Model file for the job. Use its own axes, mm. A direction names the side the tool comes from. Coordinates: 2 decimals unless noted, no trailing zeros. Loops run counter-clockwise (first coordinate to the right, second up) from the corner with the lowest first, then second, coordinate; pieces in that order, holes last.
from build123d import *

# Parameters (mm, degrees)
EXTRUDE_1_DEPTH = 15
FILLET_1_R      = 2
FILLET_2_R      = 2.5


# Read off the part's stored shape, not the designer's step: Отверстие с зазором M41
with BuildPart() as part:
    # Эскиз1 → Бобышка-Вытянуть1 (new body)
    with BuildSketch(Plane(origin=(0, 0, 0), x_dir=(1, 0, 0), z_dir=(0, 1, 0))):
        with BuildLine():
            Line((-22.5, -46.880166382), (-22.5, -45.768438907))
            ThreePointArc((-22.5, -45.768438907), (-17.354305588, -47.956522784), (-12, -49.568134926))
            Line((-12, -49.568134926), (-12, -58.568134926))
            Line((-12, -58.568134926), (12, -58.568134926))
            Line((12, -58.568134926), (12, -49.568134926))
            ThreePointArc((12, -49.568134926), (17.354305588, -47.956522784), (22.5, -45.768438907))
            Line((22.5, -45.768438907), (22.5, -46.880166382))
            ThreePointArc((22.5, -46.880166382), (17.834526239, -48.845979096), (13, -50.348783501))
            Line((13, -50.348783501), (13, -59.568134926))
            Line((13, -59.568134926), (-13, -59.568134926))
            Line((-13, -59.568134926), (-13, -50.348783501))
            ThreePointArc((-13, -50.348783501), (-17.834526239, -48.845979096), (-22.5, -46.880166382))
        make_face()
    extrude(amount=EXTRUDE_1_DEPTH)

    # Скругление1
    fillet_1_edges = [part.edges().sort_by_distance(p)[0] for p in [
        (-13, 7.5, 50.348783501),
        (13, 7.5, 50.348783501),
        (12, 7.5, 58.568134926),
        (-12, 7.5, 58.568134926),
    ]]
    fillet(fillet_1_edges, radius=FILLET_1_R)

    # Скругление2
    fillet_2_edges = [part.edges().sort_by_distance(p)[0] for p in [
        (-12, 7.5, 49.568134926),
        (-13, 7.5, 59.568134926),
        (13, 7.5, 59.568134926),
        (12, 7.5, 49.568134926),
    ]]
    fillet(fillet_2_edges, radius=FILLET_2_R)

    # Отверстие с зазором M41 outline → Отверстие с зазором M41 (revolve, cut)
    with BuildSketch(Plane(origin=(0, 8, 0), x_dir=(0.9280125149960182, 0, -0.37254901960784303), z_dir=(0, -1, 0))):
        Polygon((2.25, 52.000021479), (2.25, 51.975), (2.275021479, 52.000021479), align=None)
        Polygon((2.25, 50.950316764), (2.25, 51.975), (2.25, 52.000021479), (0, 52.000021479), (0, 50.950316764), align=None)
    revolve(axis=Axis((0, 8, 0), (0.37254901960784303, 0, 0.9280125149960182)), mode=Mode.SUBTRACT)

    # Hole Wizard M41 2 outline → Hole Wizard M41 2 (revolve, cut)
    with BuildSketch(Plane(origin=(0, 8, 0), x_dir=(0.9280125149960182, 0, 0.37254901960784303), z_dir=(0, 1, 0))):
        Polygon((2.25, -52.000019282), (2.25, -51.975), (2.25, -50.950316764), (0, -50.950316764), (0, -52.000019282), align=None)
        Polygon((2.275019282, -52.000019282), (2.249998249, -51.974998249), (2.25, -52.000019282), align=None)
    revolve(axis=Axis((0, 8, 0), (0.37254901960784303, 0, -0.9280125149960182)), mode=Mode.SUBTRACT)


solid = part.part
Q1. Slice it at C-C (y = 11). List the corners of the cut face in (x, z).
Answers:
outline: (-22.5, 45.77) arc R51 cw to (-13.82, 49.09) arc R2.5 ccw to (-12, 51.5) - (-12, 56.57) arc R2 cw to (-10, 58.57) - (10, 58.57) arc R2 cw to (12, 56.57) - (12, 51.5) arc R2.5 ccw to (13.82, 49.09) arc R51 cw to (22.5, 45.77) - (22.5, 46.88) arc R52 ccw to (14.44, 49.95) arc R2 cw to (13, 51.87) - (13, 57.07) arc R2.5 ccw to (10.5, 59.57) - (-10.5, 59.57) arc R2.5 ccw to (-13, 57.07) - (-13, 51.87) arc R2 cw to (-14.44, 49.95) arc R52 ccw to (-22.5, 46.88) - close
Q2. Drill centre lines: line 1 (X direction, y = 13.5, z = 52); line 2 (Z direction, x = 7, y = 8.5); line 3 (X direction, y = 3, z = 57.75). Where is each one in solid material? Low to high.
Answers:
line 1: x = -13 to -12, 12 to 13
line 2: z = 58.57 to 59.57
line 3: x = -12.91 to -11.61, 11.61 to 12.91
Q3. Slice it at A-A (z = 55.75). List the corners of the cut face in (x, y), and give its area (3 significant figures).
Answers:
outline: (-13, 0) - (-12, 0) - (-12, 15) - (-13, 15) - close; (12, 0) - (13, 0) - (13, 15) - (12, 15) - close
area: 30.0 mm2
Q4. Which spindle directions (+Z, -Z, +X, -X, +Y, -Y) get a long thin tool onto all of the face, cutting with end or side? Do faces 4 (the cylindrical face through (11.399, 7.605, 57.998)), 5 (the flat face through (-13, 7, 55)), 6 (the flat face through (22.5, 7, 46)), 7 (the flat face through (13, 7, 54)). Say none if no direction does.
Answers:
face 4: -Z, +Y, -Y
face 5: +Z, -X, +Y, -Y
face 6: +Z, -Z, +X, +Y, -Y
face 7: +Z, +X, +Y, -Y
Q5. Slice it at D-D (x = -1). List the corners of the cut face in (y, z).
Answers:
outline: (0, 58.57) - (15, 58.57) - (15, 59.57) - (0, 59.57) - close
Q6. Flat gauge pins, fed straight in: P1, Ø2.5, axis at y = 7.5, z = 54.5, coming from the +X side; P2, Ø5, axis at x = -7.5, z = 50.5, coming from the -Y side; P3, Ø1, axis at x = -5.5, y = 5.5, coming from the -Z side; P4, Ø1.6, axis at y = 11, z = 55, coming from the -X side. Where does each tip first touch, or does it go through?
Answers:
P1: stops at x = 13
P2: passes through
P3: stops at z = 58.57
P4: stops at x = -13
Q7. Mould opens along X. For faces 1 (the cylindrical face through (12.2, 7.6, 58.9)), 2 (the flat face through (-12, 7, 54)), 3 (the cylindrical face through (-18.48, 5.728, 48.606)) say: +X half, -X half, draft (parallel to the pull), parting line (faces both ways), or undercut.
Answers:
face 1: +X half
face 2: undercut
face 3: -X half
Q8. Slice it at B-B (y = 8.5). List the corners of the cut face in (x, z), and give its area (3 significant figures).
Answers:
outline: (-22.5, 45.77) arc R51 cw to (-21.02, 46.47) - (-21.39, 47.4) arc R52 ccw to (-22.5, 46.88) - close; (-17.32, 49.03) - (-16.95, 48.1) arc R51 cw to (-13.82, 49.09) arc R2.5 ccw to (-12, 51.5) - (-12, 56.57) arc R2 cw to (-10, 58.57) - (10, 58.57) arc R2 cw to (12, 56.57) - (12, 51.5) arc R2.5 ccw to (13.82, 49.09) arc R51 cw to (16.95, 48.1) - (17.32, 49.03) arc R52 ccw to (14.44, 49.95) arc R2 cw to (13, 51.87) - (13, 57.07) arc R2.5 ccw to (10.5, 59.57) - (-10.5, 59.57) arc R2.5 ccw to (-13, 57.07) - (-13, 51.87) arc R2 cw to (-14.44, 49.95) arc R52 ccw to start; (21.02, 46.47) arc R51 cw to (22.5, 45.77) - (22.5, 46.88) arc R52 ccw to (21.39, 47.4) - close
area: 54.3 mm2
